Verification items for the finished model (mm, model axes). Coordinates: 2 decimals unless noted, no trailing zeros. Write each loop counter-clockwise with the first axis right and the second up, starting at its lowest first coordinate (ties: lowest second). Pieces come first, ordered by that corner, then holes. Notation, with made-up numbers: (77.5, -12.75) - (115.5, -12.75) arc R20 cw to (115.5, 12.25) - close; hole circle Ø10 at (13.5, -32). An arc over 180 degrees is marked (long way). Use one line per item in the form item = value. Start each with the question number.
(1) Material ranges on line 1 (Y direction, x = 419.1, z = 3.5); line 2 (Y direction, x = 37.5, z = 4.5), recorded low to high. Write a range as [from, to].
(2) Sectioned sample at B-B (y = 158.75). Record the cut outline in (x, z) (3 decimals), and give its area (3 significant figures).
(3) Sectioned sample at C-C (z = 4.75). Record the cut outline in (x, y) (3 decimals), and give its area (3 significant figures).
(4) Gauge pin test, flat ends, axial feed: pin 1 Ø23 at (x, y) = (111.125, 158.75) entering from -Z; pin 2 Ø4 at (x, y) = (105.5, 102) entering from -Z. Record the tip position at first contact, or that the pin passes through.
(5) Sectioned sample at A-A (x = 31.75). Record the cut outline in (y, z).
(6) Mould release check, pull along Y, two halves, no side actions. Record for faces 1 (the flat face through (301, 97, 0)), 2 (the cylindrical face through (479.443, 157.912, 3.131)), 3 (the cylindrical face through (208.67, 153.03, 3.13)): released by +Y, released by -Y, zero draft, split by the parting line, or undercut.
Autodesk Inventor part; units mm, degrees
ref_plane "YZ Plane" through (0, 0, 0) normal (1, 0, 0) x (0, 1, 0)
ref_plane "XZ Plane" through (0, 0, 0) normal (0, 1, 0) x (-1, 0, 0)
ref_plane "XY Plane" through (0, 0, 0) normal (0, 0, 1) x (1, 0, 0)
sketch "Sketch1" plane through (0, 0, 0) normal (0, 0, 1) x (1, 0, 0)
  line L0 (0, 0) -> (609.6, 0)
  line L1 (609.6, 0) -> (609.6, 190.5)
  line L2 (609.6, 190.5) -> (0, 190.5)
  line L3 (0, 190.5) -> (0, 0)
  circle A0 centre (577.85, 158.75) radius 19.05
  circle A1 centre (419.1, 158.75) radius 19.05
  circle A2 centre (190.5, 158.75) radius 19.05
  circle A3 centre (31.75, 158.75) radius 19.05
  circle A4 centre (498.475, 158.75) radius 19.05
  circle A5 centre (111.125, 158.75) radius 19.05
  dimension "d0" = 190.5
  dimension "d1" = 609.6
  dimension "d13" = 38.1
  dimension "d14" = 38.1
  dimension "d15" = 228.6
  dimension "d16" = 158.75
  dimension "d17" = 79.375
  dimension "d18" = 79.375
  dimension "d21" = 31.75
  dimension "d22" = 31.75
  dimension "d23" = 31.75
extrude "Extrusion1" add sketch "Sketch1" along normal blind 6.35
equation "\"d14\" = d13"
equation "\"d16\" = 0.5 * d1 - 0.5 * d15 - d23"
equation "\"d17\" = 0.5 * d16"
equation "\"d18\" = d17"
equation "\"d23\" = d22"
properties part number "manipulator back pannel"
Answers below:
q1.line_1 = [0, 139.7], [177.8, 190.5]
q1.line_2 = [0, 140.59], [176.91, 190.5]
q2.outline = (0, 0) - (12.7, 0) - (12.7, 6.35) - (0, 6.35) - close; (50.8, 0) - (92.075, 0) - (92.075, 6.35) - (50.8, 6.35) - close; (130.175, 0) - (171.45, 0) - (171.45, 6.35) - (130.175, 6.35) - close; (209.55, 0) - (400.05, 0) - (400.05, 6.35) - (209.55, 6.35) - close; (438.15, 0) - (479.425, 0) - (479.425, 6.35) - (438.15, 6.35) - close; (517.525, 0) - (558.8, 0) - (558.8, 6.35) - (517.525, 6.35) - close; (596.9, 0) - (609.6, 0) - (609.6, 6.35) - (596.9, 6.35) - close
q2.area = 2,420 mm2
q3.outline = (0, 0) - (609.6, 0) - (609.6, 190.5) - (0, 190.5) - close; hole circle Ø38.1 at (31.75, 158.75); hole circle Ø38.1 at (111.125, 158.75); hole circle Ø38.1 at (190.5, 158.75); hole circle Ø38.1 at (419.1, 158.75); hole circle Ø38.1 at (498.475, 158.75); hole circle Ø38.1 at (577.85, 158.75)
q3.area = 109,000 mm2
q4.pin_1 = through
q4.pin_2 = 0
q5.outline = (0, 0) - (139.7, 0) - (139.7, 6.35) - (0, 6.35) - close; (177.8, 0) - (190.5, 0) - (190.5, 6.35) - (177.8, 6.35) - close
q6.face_1 = zero draft
q6.face_2 = undercut
q6.face_3 = undercut
